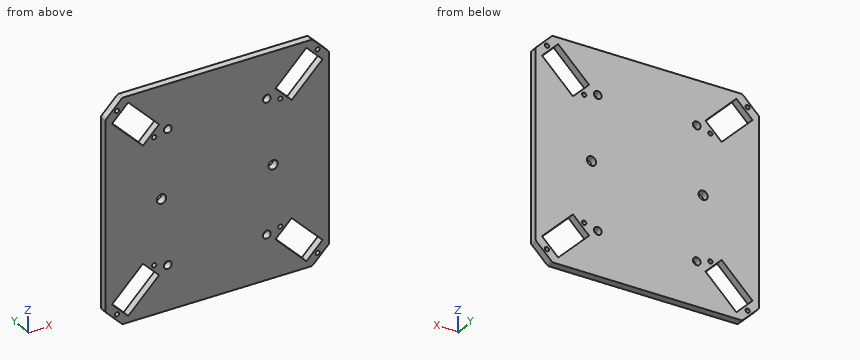
from build123d import *

# Parameters (mm, degrees)
SKETCH1_R           = 1.15
SKETCH1_R_2         = 2.5
SKETCH1_R_3         = 2.1
BOSS_EXTRUDE1_DEPTH = 4
FILLET1_R           = 1.5


with BuildPart() as part:
    # Sketch1 → Boss-Extrude1 (new body)
    with BuildSketch(Plane(origin=(0, 0, 0), x_dir=(1, 0, 0), z_dir=(0, 1, 0))):
        Polygon((-60, 51), (-60, -51), (-51, -60), (51, -60), (60, -51), (60, 51), (51, 60), (-51, 60), align=None)
        with Locations(Location((-53.918881682, 53.918881682, 0), (0, 0, 270))):
            Circle(SKETCH1_R, mode=Mode.SUBTRACT)
        with Locations(Location((-33.907759774, 33.907759774, 0), (0, 0, 270))):
            Circle(SKETCH1_R, mode=Mode.SUBTRACT)
        with Locations(Location((33.907759774, 33.907759774, 0), (0, 0, 90))):
            Circle(SKETCH1_R, mode=Mode.SUBTRACT)
        with Locations(Location((53.918881682, 53.918881682, 0), (0, 0, 90))):
            Circle(SKETCH1_R, mode=Mode.SUBTRACT)
        with Locations(Location((-53.918881682, -53.918881682, 0), (0, 0, 270))):
            Circle(SKETCH1_R, mode=Mode.SUBTRACT)
        with Locations(Location((-33.907759774, -33.907759774, 0), (0, 0, 270))):
            Circle(SKETCH1_R, mode=Mode.SUBTRACT)
        with Locations(Location((53.918881682, -53.918881682, 0), (0, 0, 90))):
            Circle(SKETCH1_R, mode=Mode.SUBTRACT)
        with Locations(Location((33.907759774, -33.907759774, 0), (0, 0, 90))):
            Circle(SKETCH1_R, mode=Mode.SUBTRACT)
        with Locations(Location((-30, 0, 0), (0, 0, 270))):
            Circle(SKETCH1_R_2, mode=Mode.SUBTRACT)
        with Locations(Location((30, 0, 0), (0, 0, 270))):
            Circle(SKETCH1_R_2, mode=Mode.SUBTRACT)
        with Locations(Location((26.599203711, 36, 0), (0, 0, 270))):
            Circle(SKETCH1_R_3, mode=Mode.SUBTRACT)
        with Locations(Location((26.599203711, -36, 0), (0, 0, 270))):
            Circle(SKETCH1_R_3, mode=Mode.SUBTRACT)
        with Locations(Location((-26.599203711, -36, 0), (0, 0, 270))):
            Circle(SKETCH1_R_3, mode=Mode.SUBTRACT)
        with Locations(Location((-26.599203711, 36, 0), (0, 0, 270))):
            Circle(SKETCH1_R_3, mode=Mode.SUBTRACT)
        Polygon((-56.570532111, 47.873118703), (-47.873118703, 56.570532111), (-31.256109345, 39.953522753), (-39.953522753, 31.256109345), align=None, mode=Mode.SUBTRACT)
        Polygon((39.953522753, 31.256109345), (31.256109345, 39.953522753), (47.873118703, 56.570532111), (56.570532111, 47.873118703), align=None, mode=Mode.SUBTRACT)
        Polygon((-47.873118703, -56.570532111), (-56.570532111, -47.873118703), (-39.953522753, -31.256109345), (-31.256109345, -39.953522753), align=None, mode=Mode.SUBTRACT)
        Polygon((47.873118703, -56.570532111), (56.570532111, -47.873118703), (39.953522753, -31.256109345), (31.256109345, -39.953522753), align=None, mode=Mode.SUBTRACT)
    extrude(amount=BOSS_EXTRUDE1_DEPTH)

    # Fillet1
    fillet1_edges = [part.edges().sort_by_distance(p)[0] for p in [
        (51, 2, -60),
        (60, 2, -51),
        (60, 2, 51),
        (51, 2, 60),
        (-51, 2, 60),
        (-60, 2, 51),
        (-60, 2, -51),
        (-51, 2, -60),
    ]]
    fillet(fillet1_edges, radius=FILLET1_R)


solid = part.part
Design review of the part built by this model. Coordinates are the model's own, in mm. Coordinates: 2 decimals unless noted, no trailing zeros. Order: outer loops, then holes, each group sorted by start corner. A loop starts at its lowest first (then second) coordinate and runs counter-clockwise, first axis right, second up. Notation, with made-up numbers: (-24.5, 18) -> (-7.5, 18) arc R30 ccw to (-7.5, 54) -> close; hole circle Ø5 at (68, 38). An arc over 180 degrees is marked (long way). Use one line per item in the form item = value. Start each with the question number.
(1) For probe 1 along X at (y, z) = (3, 0); probe 2 along Z at (x, y) = (26.5, 0.45); probe 3 along Z at (x, y) = (47, 3.7), list the stretches that pass through material, from the lowest coordinate up.
(2) Insertion check: pin 1 (3.5 mm diameter, centred on x = 26.6, z = 36, fed in from -Y); pin 2 (3 mm diameter, centred on x = 53.92, z = 53.92, fed in from -Y). Each pin has a flat end and moves straight along its axis. Give the tip position at first contact, or say it passes through.
(3) Add section A-A on z = 0. State the section outline as (x, y) points, plus the area to 3 significant figures.
(4) Add section B-B on y = 2.3. Give the number of separate pieces and of enclosed holes in the cut face, plus the area to 3 significant figures.
Answer block:
q1.probe_1 = -60 to -32.5, -27.5 to 27.5, 32.5 to 60
q1.probe_2 = -60 to -38.1, -33.9 to 33.9, 38.1 to 60
q1.probe_3 = -60 to -55.7, -38.3 to 38.3, 55.7 to 60
q2.pin_1 = through
q2.pin_2 = 0
q3.outline = (-60, 0) -> (-32.5, 0) -> (-32.5, 4) -> (-60, 4) -> close; (-27.5, 0) -> (27.5, 0) -> (27.5, 4) -> (-27.5, 4) -> close; (32.5, 0) -> (60, 0) -> (60, 4) -> (32.5, 4) -> close
q3.area = 440 mm²
q4.separate_pieces = 1
q4.enclosed_holes = 18
q4.area = 13,000 mm²
